from build123d import *

# Parameters (mm, degrees)
F0_W           = 15
F0_H           = 7
F1_DEPTH       = 35
F3_DEPTH       = 3.5
F4_SIZE        = 1.5
F6_D           = 4
F6_CSINK_D     = 8
F6_CSINK_ANGLE = 90


with BuildPart() as f1:
    # F0 (on Front) → F1 (new body, symmetric)
    with BuildSketch(Plane.XZ):
        Polygon((-23, 15), (-23, 0), (23, 0), (23, 15), (11, 15), (11, 24), (-11, 24), (-11, 15), align=None)
        with Locations((0, 17)):
            Rectangle(F0_W, F0_H, mode=Mode.SUBTRACT)
    extrude(amount=F1_DEPTH, both=True)

    # F2 (on face) → F3 (cut, through all)
    with BuildSketch(Plane.XY.offset(24)):
        with BuildLine():
            ThreePointArc((3, 15), (0, 18), (-3, 15))
            Line((-3, 15), (-3, -15))
            ThreePointArc((-3, -15), (0, -18), (3, -15))
            Line((3, -15), (3, 15))
        make_face()
    extrude(amount=-F3_DEPTH, mode=Mode.SUBTRACT)

    # F4
    f4_edges = [f1.edges().sort_by_distance(p)[0] for p in [
        (-11, 0, 15),
        (11, 0, 24),
        (-11, 0, 24),
        (11, 0, 15),
        (-23, 0, 15),
        (23, 0, 15),
    ]]
    chamfer(f4_edges, length=F4_SIZE)

    # F6 (through all)
    with Locations(Plane.XY.offset(15)):
        with Locations((17, 25), (17, -25), (-17, -25), (-17, 25)):
            CounterSinkHole(F6_D / 2, F6_CSINK_D / 2, counter_sink_angle=F6_CSINK_ANGLE)


solid = f1.part
The listing builds one solid part. Answer for the finished solid, in the listing's coordinates (mm). A direction names the side the tool comes from. Round coordinates to 2 decimals unless told otherwise and drop trailing zeros. Write each loop counter-clockwise with the first axis right and the second up, starting at its lowest first coordinate (ties: lowest second). Pieces come first, ordered by that corner, then holes. Notation, with made-up numbers: (2.5, 1.25) - (30.5, 1.25) arc R24 cw to (30.5, 35.25) - close; hole circle Ø11 at (19.25, 18). An arc over 180 degrees is marked (long way). Use one line per item in the form item = value. Start each with the question number.
Item 1: A tool of negligible diameter and unlimited length cuts with its end or side. For faces 1 (the cylindrical face through (0, -18, 22)), 2 (the flat face through (7.5, 0, 17)), 3 (the flat face through (-11, 0, 20)), 4 (the flat face through (-23, 0, 7)), from which of +Z, -Z, +X, -X, +Y, -Y can it reach the whole face along a straight path? Write none if from no direction.
Item 2: A cutting plane is placed at D-D (y = 1). Write down the section's boundary in (x, z).
Item 3: Find the intervals of material crossed by line 1 (Y direction, x = -17, z = 7.25); line 2 (X direction, y = -25, z = 8.5); line 3 (X direction, y = -19, z = 17), in increasing order. Write a range as [from, to].
Item 4: A cutting plane is placed at B-B (x = -17). Write down the section's boundary in (y, z).
Item 5: A cutting plane is placed at C-C (z = 15.75). Write down the section's boundary in (x, y), plus the area to 3 significant figures.
Item 6: A cutting plane is placed at A-A (y = -25). Give the number of separate pieces and of enclosed holes in the cut face, plus the area to 3 significant figures.
Item 7: Determine the mould class of faces 5 (the flat face through (-10.2, -0.5, 23.3)), 6 (the flat face through (11, 0, 19)), 7 (the cylindrical face through (18.6, -26.2, 6.4)) for opening direction X: +X half, -X half, draft (parallel to the pull), parting line (faces both ways), or undercut.
Item 8: Flat-ended cylindrical pins translate along their axes: pin 1 Ø1.5 at (y, z) = (-24.5, 19.5) entering from -X; pin 2 Ø2.5 at (x, y) = (-17, 25) entering from +Z; pin 3 Ø7 at (x, y) = (-19, 0) entering from +Z; pin 4 Ø3 at (x, y) = (0.5, -3.5) entering from +Z. Find the tip coordinate at first contact, or state that the pin passes through.
The answers:
q1.face_1 = +Z
q1.face_2 = +Y, -Y
q1.face_3 = +Z, -X, +Y, -Y
q1.face_4 = +Z, -Z, -X, +Y, -Y
q2.outline = (-23, 0) - (23, 0) - (23, 13.5) - (21.5, 15) - (12.5, 15) - (11, 16.5) - (11, 22.5) - (9.5, 24) - (3, 24) - (3, 20.5) - (7.5, 20.5) - (7.5, 13.5) - (-7.5, 13.5) - (-7.5, 20.5) - (-3, 20.5) - (-3, 24) - (-9.5, 24) - (-11, 22.5) - (-11, 16.5) - (-12.5, 15) - (-21.5, 15) - (-23, 13.5) - close
q3.line_1 = [-35, -27], [-23, 23], [27, 35]
q3.line_2 = [-23, -19], [-15, 15], [19, 23]
q3.line_3 = [-11, -7.5], [7.5, 11]
q4.outline = (-35, 0) - (-27, 0) - (-27, 13) - (-29, 15) - (-35, 15) - close; (-23, 0) - (23, 0) - (23, 13) - (21, 15) - (-21, 15) - (-23, 13) - close; (27, 0) - (35, 0) - (35, 15) - (29, 15) - (27, 13) - close
q5.outline = (-11.75, -35) - (-7.5, -35) - (-7.5, 35) - (-11.75, 35) - close; (7.5, -35) - (11.75, -35) - (11.75, 35) - (7.5, 35) - close
q5.area = 595 mm^2
q6.separate_pieces = 3
q6.enclosed_holes = 1
q6.area = 653 mm^2
q7.face_5 = -X half
q7.face_6 = +X half
q7.face_7 = undercut
q8.pin_1 = -11
q8.pin_2 = through
q8.pin_3 = 15
q8.pin_4 = 13.5
